```python
from build123d import *

# Parameters (mm, degrees)
F0_W      = 320.802
F0_H      = 609.6
F1_DEPTH  = 368.3
F3_DEPTH  = 609.601
F6_W      = 6.35
F6_H      = 20.32
F6_H_2    = 12.7
F8_W      = 304.8
F8_H      = 171.8733333333
F8_H_2    = 192.1933333333
F9_DEPTH  = 12.7
F11_DEPTH = 508


# Not quite as in the source:
# - a pattern or mirror of a feature is missing from the dataset's text; its kind, count and spacing are read off the source's solid


with BuildPart() as f1:
    # F0 (on Front) → F1 (new body)
    with BuildSketch(Plane.XZ):
        with Locations((160.401, 304.8)):
            Rectangle(F0_W, F0_H)
    extrude(amount=-F1_DEPTH)

    # F2 (on face) → F3 (cut, through all)
    with BuildSketch(Plane.XY.offset(609.6)):
        with BuildLine():
            ThreePointArc((160.401, 0), (79.2011834962, 6.3893162785), (0, 25.4))
            Line((0, 25.4), (0, 0))
            Line((0, 0), (160.401, 0))
        make_face()
        with BuildLine():
            Line((320.802, 0), (320.802, 25.4))
            ThreePointArc((320.802, 25.4), (241.6008165038, 6.3893162785), (160.401, 0))
            Line((160.401, 0), (320.802, 0))
        make_face()
    extrude(amount=-F3_DEPTH, mode=Mode.SUBTRACT)

    # F6 (on mid) → F7 (revolve, cut)
    with BuildSketch(Plane.YZ.offset(160.401)):
        with Locations((3.175, 599.44)):
            Rectangle(F6_W, F6_H)
        with Locations((3.175, 407.2466666667)):
            Rectangle(F6_W, F6_H)
        with Locations((3.175, 215.0533333333)):
            Rectangle(F6_W, F6_H)
        with Locations((3.175, 6.35)):
            Rectangle(F6_W, F6_H_2)
    revolve(axis=Axis((160.401, 519.1661575, 538.612387991), (0, 0, -1)), mode=Mode.SUBTRACT)

    # F8 (on face) → F9 (cut)
    with BuildSketch(Plane.YZ.offset(320.802)):
        with Locations((196.85, 503.3433333333)):
            Rectangle(F8_W, F8_H)
        with Locations((196.85, 311.15)):
            Rectangle(F8_W, F8_H)
        with Locations((196.85, 108.7966666667)):
            Rectangle(F8_W, F8_H_2)
    f9 = extrude(amount=-F9_DEPTH, mode=Mode.SUBTRACT)

    # F9_copies: F9 across plane
    add(f9.mirror(Plane(origin=(160.401, 0, 0), x_dir=(0, 0, -1), z_dir=(-1, 0, 0))), mode=Mode.SUBTRACT)

    # F10 (on face) → F11 (cut)
    with BuildSketch(Plane(origin=(0, 0, 0), x_dir=(1, 0, 0), z_dir=(0, 0, -1))):
        with BuildLine():
            Line((101.6, -266.7), (219.202, -266.7))
            Line((219.202, -266.7), (219.202, -112.1757760558))
            ThreePointArc((219.202, -112.1757760558), (160.401, -107.95), (101.6, -112.1757760558))
            Line((101.6, -112.1757760558), (101.6, -266.7))
        make_face()
    extrude(amount=-F11_DEPTH, mode=Mode.SUBTRACT)


solid = f1.part
```
For this review, take the finished solid that the model builds, in its own axes (mm). A direction names the side the tool comes from. Coordinates: 2 decimals unless noted, no trailing zeros. Order: outer loops, then holes, each group sorted by start corner. A loop starts at its lowest first (then second) coordinate and runs counter-clockwise, first axis right, second up. Notation, with made-up numbers: (25.25, 89.5) -> (63.25, 89.5) arc R20 ccw to (63.25, 120.5) -> close; hole circle Ø10 at (-17.75, -2). An arc over 180 degrees is marked (long way). Answer as CSV lines item,"result".
Q1. For faces 4 (the face through (308.102, 195, 505)), 5 (the face through (160, 5, 417.407)), 6 (the face through (6, 349.25, 107)), list the 3-axis set-ups (+Z, -Z, +X, -X, +Y, -Y) from which the entire face can be reached by the end or side of a thin tool; tool diameter is ignored.
Model answer:
face 4,"+X"
face 5,"-Y"
face 6,"-X"
Q2. Wall thickness on line 1 along X through (y, z) = (148, 367); line 2 along Y through (x, z) = (170, 171.5); line 3 along X through (y, z) = (255.5, 399.5): over which ranges is each line inside the solid? List them lowest first. Write a range as [from, to].
Model answer:
line 1,"x = [12.7, 101.6], [219.2, 308.1]"
line 2,"y = [0.09, 108.06], [266.7, 368.3]"
line 3,"x = [0, 101.6], [219.2, 320.8]"
Q3. We need section C-C (x = 276). State the section outline as (y, z) points.
Model answer:
outline,"(13.03, 12.7) -> (19.55, 12.7) -> (19.55, 0) -> (368.3, 0) -> (368.3, 609.6) -> (19.55, 609.6) -> (19.55, 589.28) -> (13.03, 589.28) -> (13.03, 417.41) -> (19.55, 417.41) -> (19.55, 397.09) -> (13.03, 397.09) -> (13.03, 225.21) -> (19.55, 225.21) -> (19.55, 204.89) -> (13.03, 204.89) -> close"
Q4. Clearance check with flat-ended pins moving along their axes: pin 1 Ø14 at (x, y) = (314, 250) entering from -Z; pin 2 Ø2 at (x, z) = (60, 156) entering from -Y; pin 3 Ø2 at (x, y) = (157.5, 125) entering from -Z; pin 4 Ø6.5 at (x, z) = (7.5, 64) entering from -Y. State where each tip first meets the part, or that it passes through.
Model answer:
pin 1,"stops at z = 0"
pin 2,"stops at y = 9.6"
pin 3,"stops at z = 508"
pin 4,"stops at y = 22.04"
Q5. We need section D-D (z = 519). State the section outline as (x, y) points.
Model answer:
outline,"(0, 25.4) arc R519.17 ccw to (320.8, 25.4) -> (320.8, 44.45) -> (308.1, 44.45) -> (308.1, 349.25) -> (320.8, 349.25) -> (320.8, 368.3) -> (0, 368.3) -> (0, 349.25) -> (12.7, 349.25) -> (12.7, 44.45) -> (0, 44.45) -> close"
Q6. We need section B-B (y = 332). State the section outline as (x, z) points.
Model answer:
outline,"(0, 0) -> (320.8, 0) -> (320.8, 12.7) -> (308.1, 12.7) -> (308.1, 204.89) -> (320.8, 204.89) -> (320.8, 225.21) -> (308.1, 225.21) -> (308.1, 397.09) -> (320.8, 397.09) -> (320.8, 417.41) -> (308.1, 417.41) -> (308.1, 589.28) -> (320.8, 589.28) -> (320.8, 609.6) -> (0, 609.6) -> (0, 589.28) -> (12.7, 589.28) -> (12.7, 417.41) -> (0, 417.41) -> (0, 397.09) -> (12.7, 397.09) -> (12.7, 225.21) -> (0, 225.21) -> (0, 204.89) -> (12.7, 204.89) -> (12.7, 12.7) -> (0, 12.7) -> close"
Q7. We need section A-A (z = 73). State the section outline as (x, y) points.
Model answer:
outline,"(0, 25.4) arc R519.17 ccw to (320.8, 25.4) -> (320.8, 44.45) -> (308.1, 44.45) -> (308.1, 349.25) -> (320.8, 349.25) -> (320.8, 368.3) -> (0, 368.3) -> (0, 349.25) -> (12.7, 349.25) -> (12.7, 44.45) -> (0, 44.45) -> close; hole (101.6, 112.18) arc R411.22 ccw to (219.2, 112.18) -> (219.2, 266.7) -> (101.6, 266.7) -> close"
Q8. Draft analysis for pull direction Y (two halves, no side actions). For faces 1 (the face through (320.802, 171, 213)), 2 (the face through (160, 186, 508)), 3 (the face through (162.685, 6.355, 215.196)), state which applies: released by +Y, released by -Y, zero draft, split by the parting line, or undercut.
Model answer:
face 1,"zero draft"
face 2,"undercut"
face 3,"released by -Y"
